The model under review builds one solid part; all positions refer to its coordinate system, in mm. A direction names the side the tool comes from. Coordinates: 2 decimals unless noted, no trailing zeros. Order: outer loops, then holes, each group sorted by start corner. A loop starts at its lowest first (then second) coordinate and runs counter-clockwise, first axis right, second up. Notation, with made-up numbers: (-39.5, 21) -> (-28.5, 21) arc R27 cw to (-28.5, 48) -> close; hole circle Ø2 at (-7.5, -26.5). An arc over 180 degrees is marked (long way). Put each result on its own line as item: value.
from build123d import *

# Parameters (mm, degrees)
SKETCH_1_R          = 4.5
SKETCH_1_R_2        = 2
EXTRUDE_1_DEPTH     = 2.5
SKETCH_2_R          = 5.15
SKETCH_2_R_2        = 2
EXTRUDE_2_DEPTH     = 0.6
SKETCH_4_R          = 4
SKETCH_4_R_2        = 2.5
CUT_EXTRUDE_1_DEPTH = 0.2


with BuildPart() as part:
    # 草图1 → 凸台-拉伸1 (new body)
    with BuildSketch(Plane(origin=(0, 0, 0), x_dir=(1, 0, 0), z_dir=(0, 1, 0))):
        with Locations(Location((0, 0, 0), (0, 0, 270))):
            Circle(SKETCH_1_R)
        with Locations(Location((0, 0, 0), (0, 0, 270))):
            Circle(SKETCH_1_R_2, mode=Mode.SUBTRACT)
    extrude(amount=EXTRUDE_1_DEPTH)

    # 草图2 → 凸台-拉伸2 (add)
    with BuildSketch(Plane.XZ):
        with Locations(Location((0, 0, 0), (0, 0, 270))):
            Circle(SKETCH_2_R)
        with Locations(Location((0, 0, 0), (0, 0, 90))):
            Circle(SKETCH_2_R_2, mode=Mode.SUBTRACT)
    extrude(amount=-EXTRUDE_2_DEPTH)

    # 草图4 → 切除-拉伸1 (cut)
    with BuildSketch(Plane(origin=(0, 2.5, 0), x_dir=(1, 0, 0), z_dir=(0, 1, 0))):
        with Locations(Location((0, 0, 0), (0, 0, 270))):
            Circle(SKETCH_4_R)
        with Locations(Location((0, 0, 0), (0, 0, 270))):
            Circle(SKETCH_4_R_2, mode=Mode.SUBTRACT)
    cut_extrude_1 = extrude(amount=-CUT_EXTRUDE_1_DEPTH, mode=Mode.SUBTRACT)

    # 镜向1: 切除-拉伸1 across plane
    add(cut_extrude_1.mirror(Plane(origin=(0, 1.25, 0), x_dir=(0, 0, 1), z_dir=(0, -1, 0))), mode=Mode.SUBTRACT)


solid = part.part
Item 1: Mouldability with a two-part tool opening along X and no side actions: class faces 1 (the flat face through (2, 2.5, -1)), 2 (the flat face through (2, 0.2, 2)), 3 (the cylindrical face through (1.352, 1.537, 4.292)), 4 (the flat face through (2, 2.3, 2)) as +X half, -X half, draft (parallel to the pull), parting line (faces both ways), or undercut.
Answers below:
face 1: draft
face 2: undercut
face 3: parting line
face 4: undercut
Item 2: For pin 1 Ø1.5 at (x, z) = (1.5, -0.5) entering from +Y; pin 2 Ø1 at (x, y) = (1.5, 1) entering from -Z, all flat-tipped, find the tip position at first contact; note any pin that passes through.
Answers below:
pin 1: y = 2.5
pin 2: z = -5.01
Item 3: Consider section C-C on y = 0.9. Write out the cut boundary in (x, z).
Answers below:
outline: circle Ø9 at (0, 0); hole circle Ø4 at (0, 0)
Item 4: Consider section B-B on x = 0. Write out the cut boundary in (y, z), and give its area (3 significant figures).
Answers below:
outline: (0, -5.15) -> (0.6, -5.15) -> (0.6, -4.5) -> (2.5, -4.5) -> (2.5, -4) -> (2.3, -4) -> (2.3, -2.5) -> (2.5, -2.5) -> (2.5, -2) -> (0, -2) -> (0, -2.5) -> (0.2, -2.5) -> (0.2, -4) -> (0, -4) -> close; (0, 2) -> (2.5, 2) -> (2.5, 2.5) -> (2.3, 2.5) -> (2.3, 4) -> (2.5, 4) -> (2.5, 4.5) -> (0.6, 4.5) -> (0.6, 5.15) -> (0, 5.15) -> (0, 4) -> (0.2, 4) -> (0.2, 2.5) -> (0, 2.5) -> close
area: 12.1 mm^2
Item 5: For line 1 (X direction, y = 2.4, z = 0); line 2 (X direction, y = 0.9, z = 0); line 3 (Y direction, x = 4.75, z = -1.5), list the stretches that pass through material, from the lowest coordinate up. Write a range as from..to.
Answers below:
line 1: -4.5..-4, -2.5..-2, 2..2.5, 4..4.5
line 2: -4.5..-2, 2..4.5
line 3: 0..0.6
Item 6: Consider section A-A on z = 0. Write out the cut boundary in (x, y), and give its area (3 significant figures).
Answers below:
outline: (-5.15, 0) -> (-4, 0) -> (-4, 0.2) -> (-2.5, 0.2) -> (-2.5, 0) -> (-2, 0) -> (-2, 2.5) -> (-2.5, 2.5) -> (-2.5, 2.3) -> (-4, 2.3) -> (-4, 2.5) -> (-4.5, 2.5) -> (-4.5, 0.6) -> (-5.15, 0.6) -> close; (2, 0) -> (2.5, 0) -> (2.5, 0.2) -> (4, 0.2) -> (4, 0) -> (5.15, 0) -> (5.15, 0.6) -> (4.5, 0.6) -> (4.5, 2.5) -> (4, 2.5) -> (4, 2.3) -> (2.5, 2.3) -> (2.5, 2.5) -> (2, 2.5) -> close
area: 12.1 mm^2
Item 7: For faces 5 (the flat face through (-5, 0.6, 0)), 6 (the cylindrical face through (-2, 1, 0)), list the 3-axis set-ups (+Z, -Z, +X, -X, +Y, -Y) from which the entire face can be reached by the end or side of a thin tool; tool diameter is ignored.
Answers below:
face 5: +Y
face 6: +Y, -Y
Item 8: Consider section D-D on x = -3.75. Write out the cut boundary in (y, z).
Answers below:
outline: (0, -3.53) -> (0.6, -3.53) -> (0.6, -2.49) -> (2.5, -2.49) -> (2.5, -1.39) -> (2.3, -1.39) -> (2.3, 1.39) -> (2.5, 1.39) -> (2.5, 2.49) -> (0.6, 2.49) -> (0.6, 3.53) -> (0, 3.53) -> (0, 1.39) -> (0.2, 1.39) -> (0.2, -1.39) -> (0, -1.39) -> close
